Could you check a few things on this model? Use its own coordinates, in mm. Face numbers are marked on the shaded views. A direction names the side the tool comes from. Round coordinates to 2 decimals unless told otherwise and drop trailing zeros. Write each loop counter-clockwise with the first axis right and the second up, starting at its lowest first coordinate (ties: lowest second). Pieces come first, ordered by that corner, then holes. Notation, with made-up numbers: (45, 78) - (87, 78) arc R26 cw to (87, 114) - close; hole circle Ø1 at (-10, -40). An arc over 180 degrees is marked (long way). Write each question's results on one line, items separated by ' | '. Start each with the question number.
(1) Imagine slicing it at C-C on y = 8.25. State how many separate pieces and enclosed holes the cut face has, then the cut area to 3 significant figures.
(2) Imagine slicing it at A-A on z = 0.75. Write out the boundary of the cut face in (x, y).
(3) Imagine slicing it at B-B on x = 15.5. Write out the boundary of the cut face in (y, z), then the cut area to 3 significant figures.
(4) Please list where these lines run through material, in increasing order: line 1 (Z direction, x = 0, y = 5); line 2 (X direction, y = 1.75, z = -35.75); line 3 (Z direction, x = -15.5, y = 4). Write a range as [from, to].
(5) For P1, Ø11, axis at x = 0, z = 28.25, coming from the -Y side; P2, Ø7, axis at x = -29, z = -35.75, coming from the +Y side, each with a flat end and sliding along its axis, tell me the tip position at first contact or that it passes through.
(6) On a 3-axis mill with a long thin cutter (end or side, diameter ignored), from which of +Z, -Z, +X, -X, +Y, -Y can I reach the whole of each face in a straight line? I mean the marked faces 1, 2 and 3. Say none if no direction works.
(7) Thinking about a two-plate mould opening in X: for the marked faces 4, 5, 6 and 7, which applies, +X half, -X half, draft (parallel to the pull), parting line (faces both ways), or undercut?
(8) Imagine slicing it at D-D on z = 15.5. Write out the boundary of the cut face in (x, y), then the cut area to 3 significant figures.
Solid Edge part; units mm, degrees
sketch "Sketch1" plane through (0, 0, 0) normal (0, -1, 0) x (1, 0, 0)
  line L0 (-34, -45.75) -> (34, -45.75)
  line L1 (34, -45.75) -> (34, 45.75)
  line L2 (34, 45.75) -> (-34, 45.75)
  line L3 (-34, 45.75) -> (-34, -45.75)
  dimension "D1" = 34
  dimension "D2" = 34
extrude "Protrusion1" add sketch "Sketch1" against normal blind 12
sketch "Sketch2" plane through (0, 0, 0) normal (0, -1, 0) x (1, 0, 0)
  circle A0 centre (0, -14.75) radius 11.25
  circle A1 centre (-15.5, 0.75) radius 1.7
  circle A2 centre (-15.5, -30.25) radius 1.7
  circle A3 centre (15.5, -30.25) radius 1.7
  circle A4 centre (15.5, 0.75) radius 1.7
extrude "Cutout1" cut sketch "Sketch2" against normal through all
sketch "Sketch3" plane through (0, 0, 0) normal (0, -1, 0) x (1, 0, 0)
  circle A0 centre (8.4853, 36.7353) radius 1.4
  circle A1 centre (8.4853, 19.7647) radius 1.4
  circle A2 centre (-8.4853, 19.7647) radius 1.4
  circle A3 centre (-8.4853, 36.7353) radius 1.4
  circle A4 centre (0, 28.25) radius 6
  dimension "D1" = 8.4853
extrude "Cutout2" cut sketch "Sketch3" against normal through all
sketch "Sketch4" plane through (-34, 6, 0) normal (-1, 0, 0) x (0, 0, -1)
  line L0 (-19.89, -6) -> (45.75, -71.64)
  line L1 (45.75, -71.64) -> (45.75, -6)
  line L2 (45.75, -6) -> (-19.89, -6)
extrude "Extrusionsausprägung_2" add sketch "Sketch4" against normal blind 10
mirror "Mirror1" about plane through (0, 0, 0) normal (1, 0, 0) of "Extrusionsausprägung_2"
sketch "Sketch5" plane through (-34, 38.82, 0) normal (-1, 0, 0) x (0, 0, -1)
  circle A0 centre (33.7465, 1.4635) radius 1.875
  circle A1 centre (19.6043, 15.6057) radius 1.875
  dimension "D1" = 19.6043
extrude "Extrusionsausschnitt_3" cut sketch "Sketch5" against normal blind 14
sketch "Sketch6" plane through (-34, 38.82, 0) normal (-1, 0, 0) x (0, 0, -1)
  line L0 (45.75, -38.82) -> (-31.89, 38.82)
  line L1 (-31.89, 38.82) -> (-17.75, 38.82)
  line L2 (-17.75, 38.82) -> (45.75, -24.68)
  line L3 (45.75, -24.68) -> (45.75, -38.82)
  dimension "D1" = 31.89
extrude "Extrusionsausprägung_4" add sketch "Sketch6" along normal blind 44
mirror "Mirror2" about plane through (0, 0, 0) normal (1, 0, 0) of "Extrusionsausprägung_4"
sketch "Sketch7" plane through (-54, 31.75, -14) normal (0, -0.7071068, -0.7071068) x (1, 0, 0)
  circle A0 centre (-14, 10.2613) radius 4
  circle A1 centre (-14, -19.7387) radius 4
extrude "Cutout3" cut sketch "Sketch7" against normal up to next
mirror "Mirror3" about plane through (0, 0, 0) normal (1, 0, 0) of "Cutout3"
sketch "Sketch8" plane through (-78, 38.82, -6.93) normal (-1, 0, 0) x (0, 0.7071068, -0.7071068)
  line L0 (29.953, 0) -> (42.4264, 12.4734)
extrude "Cutout4" cut sketch "Sketch8" against normal through all material side at (-78, 60.05, -36.93)
sketch "Sketch9" plane through (78, 30, -5.18) normal (1, 0, 0) x (0, -0.7071068, 0.7071068)
  line L0 (30.4551, -4.9992) -> (47.4257, -4.9992)
  line L1 (47.4257, -4.9992) -> (57.2262, -14.7997)
  line L2 (57.2262, -14.7997) -> (48.7409, -23.285)
  line L3 (48.7409, -23.285) -> (30.4551, -4.9992)
extrude "Extrusionsausschnitt_6" cut sketch "Sketch9" against normal blind 55
mirror "Mirror4" about plane through (0, 0, 0) normal (1, 0, 0) of "Extrusionsausschnitt_6"
fillet "Verrundung_1" radius 5 4 edges at (23, 6, 45.75) (-23, 6, 45.75) (34, 30, -45.75) (-34, 30, -45.75)
chamfer "Chamfer1" distance 0.5 angle 45 2 edges at (-34, 23.2143, -17.7293) (-34, 37.3565, -31.8715)
chamfer "Fase_2" distance 0.4 angle 45 4 edges at (-17.2, 0, -30.25) (-17.2, 0, 0.75) (13.8, 0, 0.75) (13.8, 0, -30.25)
chamfer "Fase_3" distance 0.4 angle 45 4 edges at (-9.8853, 0, 19.7647) (-9.8853, 0, 36.7353) (7.0853, 0, 36.7353) (7.0853, 0, 19.7647)
chamfer "Fase_4" distance 2.5 angle 45 2 edges at (-11.25, 0, -14.75) (0, 12, -3.5)
chamfer "Fase_5" distance 1.4 angle 45 2 edges at (-6, 0, 28.25) (0, 12, 34.25)
chamfer "Fase_7" distance 1 angle 45 4 edges at (-68, 34.3926, -2.5026) (-68, 55.6058, -23.7158) (68, 34.3926, -2.5026) (68, 55.6058, -23.7158)
sketch "Sketch10" plane through (-78, 30, -5.18) normal (-1, 0, 0) x (0, 0.7071068, -0.7071068)
  line L0 (-30.4551, -4.9992) -> (-20.4566, 4.9992)
extrude "Extrusionsausschnitt_8" cut sketch "Sketch10" against normal blind 44 material side at (-78, 11.95, 12.82)
mirror "Mirror5" about plane through (0, 0, 0) normal (1, 0, 0) of "Extrusionsausschnitt_8"
sketch "Sketch11" plane through (-78, 36, -11.18) normal (-1, 0, 0) x (0, 0.7071068, -0.7071068)
  line L0 (-38.9404, -4.9992) -> (7.4741, 41.4152)
extrude "Cutout6" cut sketch "Sketch11" against normal through all material side at (-78, 12.05, -12.93)
sketch "Sketch12" plane through (0, 0, 0) normal (0, -1, 0) x (0, 0, -1)
  circle A0 centre (35.75, -29) radius 2.25
  circle A1 centre (11.75, -29) radius 2.25
  circle A2 centre (-12.25, -29) radius 2.25
  dimension "D1" = 35.75
extrude "Cutout7" cut sketch "Sketch12" against normal through all
mirror "Mirror6" about plane through (0, 0, 0) normal (1, 0, 0) of "Cutout7"
sketch "Sketch13" plane through (0, 6, -45.75) normal (0, 0, -1) x (1, 0, 0)
  line L0 (-34, -6) -> (-24, -6)
  line L1 (-24, -6) -> (-24, -1)
  line L2 (-24, -1) -> (-34, -1)
  line L3 (-34, -1) -> (-34, -6)
  dimension "D1" = 34
  dimension "D2" = 34
extrude "Cutout8" cut sketch "Sketch13" against normal through all
mirror "Mirror7" about plane through (0, 0, 0) normal (1, 0, 0) of "Cutout8"
properties material "Nylon, allgemein"
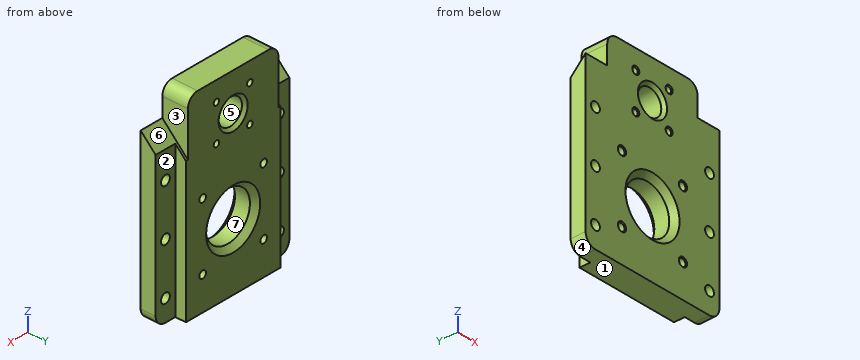
Response:
1) separate pieces: 1 | enclosed holes: 10 | area: 3,770 mm²
2) outline: (-34, 0) - (-17.6, 0) - (-17.2, 0.4) - (-17.2, 12) - (-24, 12) - (-24, 7) - (-34, 7) - close; (-13.8, 0.4) - (-13.4, 0) - (13.4, 0) - (13.8, 0.4) - (13.8, 12) - (-13.8, 12) - close; (17.2, 0.4) - (17.6, 0) - (34, 0) - (34, 7) - (24, 7) - (24, 12) - (17.2, 12) - close
3) outline: (0, -45.75) - (12, -45.75) - (12, -31.95) - (0.4, -31.95) - (0, -32.35) - close; (0, -28.15) - (0.4, -28.55) - (12, -28.55) - (12, -0.95) - (0.4, -0.95) - (0, -1.35) - close; (0, 2.85) - (0.4, 2.45) - (12, 2.45) - (12, 45.75) - (0, 45.75) - close | area: 1,020 mm²
4) line 1: [-45.75, -26], [-3.5, 22.25], [34.25, 45.75] | line 2: [-34, -31.25], [-26.75, 26.75], [31.25, 34] | line 3: [-45.75, -31.95], [-28.55, -0.95], [2.45, 45.75]
5) P1: through | P2: y = 7
6) face 1: -Z, +X, -X, +Y, -Y | face 2: +Z, -Z, +X, +Y | face 3: +Z, +X, +Y
7) face 4: -X half | face 5: undercut | face 6: draft | face 7: undercut
8) outline: (-34, 0) - (34, 0) - (34, 7) - (24, 7) - (24, 12) - (-24, 12) - (-24, 7) - (-34, 7) - close | area: 716 mm²
